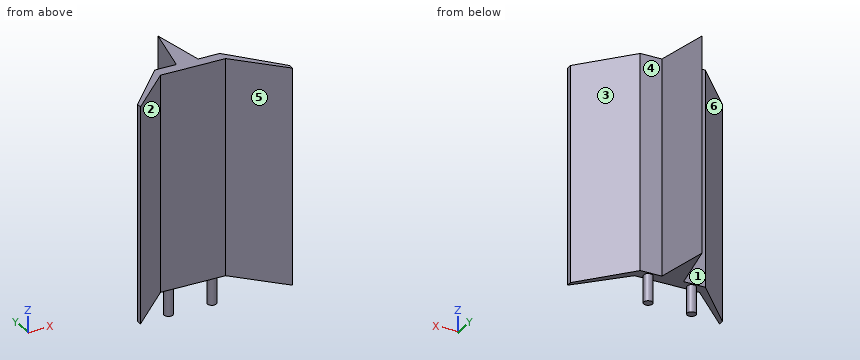
```python
from build123d import *

# Parameters (mm, degrees)
F0_R     = 2.54
F1_DEPTH = 127
F2_DEPTH = 15.875


with BuildPart() as f1:
    # F0 (on Top) → F1 (new body)
    with BuildSketch(Plane.XY):
        Polygon((-19.05, 0), (0, 0), (19.05, 0), (44.45, -25.4), (44.45, -22.225), (19.05, 6.35), (6.35, 6.35), (0, 38.1), (-6.35, 6.35), (-19.05, 6.35), (-44.45, -22.225), (-44.45, -25.4), align=None)
        with Locations((-12.7, 3.175)):
            Circle(F0_R, mode=Mode.SUBTRACT)
        with Locations((12.7, 3.175)):
            Circle(F0_R, mode=Mode.SUBTRACT)
        with Locations((-12.7, 3.175)):
            Circle(F0_R)
        with Locations((12.7, 3.175)):
            Circle(F0_R)
    extrude(amount=F1_DEPTH)

    # F0 (on Top) → F2 (join)
    with BuildSketch(Plane.XY):
        with Locations((-12.7, 3.175)):
            Circle(F0_R)
        with Locations((12.7, 3.175)):
            Circle(F0_R)
    extrude(amount=-F2_DEPTH)


solid = f1.part
```
Model file for the job. Use its own axes, mm. Face numbers are marked on the shaded views. A direction names the side the tool comes from. Give positions to 0.01 mm unless a question says otherwise; leave off trailing zeros. Order: outer loops, then holes, each group sorted by start corner. A loop starts at its lowest first (then second) coordinate and runs counter-clockwise, first axis right, second up.
1) Mould opens along X. For the marked faces 4, 5 and 6 say: +X half, -X half, draft (parallel to the pull), parting line (faces both ways), or undercut.
2) Saw through at D-D, the plane y = 19.5. Write the cut outline in (x, z).
3) Saw through at A-A, the plane y = -15.5. Write the cut outline in (x, z), then the cut area to 3 significant figures.
4) Saw through at B-B, the plane z = 80.5. Write the cut outline in (x, y) (3 decimals), then the cut area to 3 significant figures.
5) Saw through at C-C, the plane x = 12.7. Write the cut outline in (y, z) (3 decimals), then the cut area to 3 significant figures.
6) 3-axis set-ups, long thin cutter, end or side, ignore diameter. For the marked faces 1, 2 and 3: which of +Z, -Z, +X, -X, +Y, -Y reach the whole face in a straight line?
7) Wall check: probe 1 along Y at (x, z) = (-7.5, 23.5); probe 2 along X at (y, z) = (-2, 25); probe 3 along X at (y, z) = (10.5, 108). Give the ranges that are in metal, low to high.
8) Pin check, flat tips, straight feed: pin 1 (6.5 mm diameter, centred on x = 11, z = 80.5, fed in from +Y); pin 2 (3 mm diameter, centred on y = 31, z = 15, fed in from -X); pin 3 (12 mm diameter, centred on y = 0, z = 98, fed in from -X). Stop position of each tip, or through.
Computed:
1. face 4: draft
1. face 5: undercut
1. face 6: -X half
2. outline: (-3.72, 0) - (3.72, 0) - (3.72, 127) - (-3.72, 127) - close
3. outline: (-38.47, 0) - (-34.55, 0) - (-34.55, 127) - (-38.47, 127) - close; (34.55, 0) - (38.47, 0) - (38.47, 127) - (34.55, 127) - close
3. area: 996 mm2
4. outline: (-44.45, -25.4) - (-19.05, 0) - (19.05, 0) - (44.45, -25.4) - (44.45, -22.225) - (19.05, 6.35) - (6.35, 6.35) - (0, 38.1) - (-6.35, 6.35) - (-19.05, 6.35) - (-44.45, -22.225) - close
4. area: 685 mm2
5. outline: (0, 0) - (0.635, 0) - (0.635, -15.875) - (5.715, -15.875) - (5.715, 0) - (6.35, 0) - (6.35, 127) - (0, 127) - close
5. area: 887 mm2
6. face 1: +Z, -Z, -X, +Y
6. face 2: +Z, -Z, -Y
6. face 3: +Z, -Z, +X, +Y
7. probe 1: y = 0 to 6.35
7. probe 2: x = -26.47 to -21.05, 21.05 to 26.47
7. probe 3: x = -5.52 to 5.52
8. pin 1: stops at y = 6.35
8. pin 2: stops at x = -1.72
8. pin 3: stops at x = -30.03
